```python
from build123d import *

# Parameters (mm, degrees)
F1_DEPTH = 42


with BuildPart() as f1:
    # F0 (on Right) → F1 (new body)
    with BuildSketch(Plane.YZ):
        with BuildLine():
            Line((2.25, 10), (6.75, 10))
            Line((6.75, 10), (6.75, 14.565794))
            ThreePointArc((6.75, 14.565794), (6.622824, 14.872824), (6.315794, 15))
            Line((6.315794, 15), (2.684206, 15))
            ThreePointArc((2.684206, 15), (2.377176, 14.872824), (2.25, 14.565794))
            Line((2.25, 14.565794), (2.25, 10))
        make_face()
        with BuildLine():
            Line((2.25, 5.776099), (2.25, 0.066271))
            add(Edge.make_bspline(
                [(2.25, 0.066271), (2.301244, 1.931495), (6.745765, 0.11442), (6.75, 10)],
                knots=[0.125472, 0.125472, 0.125472, 0.125472, 10.965856, 10.965856, 10.965856, 10.965856], degree=3))
            Line((6.75, 10), (2.25, 10))
            Line((2.25, 10), (2.25, 5.776099))
        make_face()
        with BuildLine():
            ThreePointArc((-2.25, -9.565794), (-2.122824, -9.872824), (-1.815794, -10))
            Line((-1.815794, -10), (1.815794, -10))
            ThreePointArc((1.815794, -10), (2.122824, -9.872824), (2.25, -9.565794))
            Line((2.25, -9.565794), (2.25, 0))
            add(Edge.make_bspline(
                [(2.25, 0), (2.249402, 0.022599), (2.249407, 0.044682), (2.25, 0.066271)],
                knots=[0, 0, 0, 0, 0.125472, 0.125472, 0.125472, 0.125472], degree=3))
            Line((2.25, 0.066271), (2.25, 5.776099))
            Line((2.25, 5.776099), (-2.25, 5.776099))
            Line((-2.25, 5.776099), (-2.25, 0.066271))
            add(Edge.make_bspline(
                [(-2.25, 0), (-2.249402, 0.022599), (-2.249407, 0.044682), (-2.25, 0.066271)],
                knots=[0, 0, 0, 0, 0.125472, 0.125472, 0.125472, 0.125472], degree=3))
            Line((-2.25, 0), (-2.25, -9.565794))
        make_face()
        with BuildLine():
            add(Edge.make_bspline(
                [(-2.25, 0.066271), (-2.301244, 1.931495), (-6.745765, 0.11442), (-6.75, 10)],
                knots=[0.125472, 0.125472, 0.125472, 0.125472, 10.965856, 10.965856, 10.965856, 10.965856], degree=3))
            Line((-2.25, 0.066271), (-2.25, 5.776099))
            Line((-2.25, 5.776099), (-2.25, 10))
            Line((-2.25, 10), (-6.75, 10))
        make_face()
        with BuildLine():
            Line((-6.75, 14.565794), (-6.75, 10))
            Line((-6.75, 10), (-2.25, 10))
            Line((-2.25, 10), (-2.25, 14.565794))
            ThreePointArc((-2.25, 14.565794), (-2.377176, 14.872824), (-2.684206, 15))
            Line((-2.684206, 15), (-6.315794, 15))
            ThreePointArc((-6.315794, 15), (-6.622824, 14.872824), (-6.75, 14.565794))
        make_face()
    extrude(amount=F1_DEPTH)


solid = f1.part
```
For this review, take the finished solid that the model builds, in its own axes (mm). A direction names the side the tool comes from. Round coordinates to 2 decimals unless told otherwise and drop trailing zeros. Write each loop counter-clockwise with the first axis right and the second up, starting at its lowest first coordinate (ties: lowest second). Pieces come first, ordered by that corner, then holes. Notation, with made-up numbers: M 35,-21.5 L 89,-21.5 A34 ccw 89,17.5 Z; hole C -21.75,69 d4. An arc over 180 degrees is marked long. One line per item, written item: value. Start each with the question number.
(1) We need section A-A (z = 12). Give the boundary of the cut face in (x, y), and give its area (3 significant figures).
(2) Wall thickness on line 1 (Y direction, x = 10.5, z = 12); line 2 (Z direction, x = 16, y = -1); line 3 (Y direction, x = 34.5, z = -4): over which ranges is each line inside the solid? List them lowest first.
(3) Insertion check: pin 1 (3 mm diameter, centred on x = 26.5, z = -6, fed in from -Y); pin 2 (8 mm diameter, centred on y = 5, z = 2.5, fed in from +X); pin 3 (1.5 mm diameter, centred on x = 37.5, z = 6.5, fed in from -Y); pin 4 (12 mm diameter, centred on x = 10.5, z = 3, fed in from -Y). Each pin has a flat end and moves straight along its axis. Give the tip position at first contact, or say it passes through.
(4) The part is to be moulded in two halves that separate along Y. For faces 1 (the flat face through (0, 0, 5)), 2 (the flat face through (21, 2.25, -5)), 3 (the flat face through (21, 0, 5.776)), say which applies: released by +Y, released by -Y, zero draft, split by the parting line, or undercut.
(5) Machinability: for faces 4 (the flat face through (21, -2.25, 10)), 5 (the flat face through (21, -2.25, -5)), 6 (the flat face through (21, 0, -10)), which of the approach directions +Z, -Z, +X, -X, +Y, -Y give a long, thin tool a straight path to every point of the face, cutting with its end or side? Answer none if there is none.
Result:
1. outline: M 0,-6.75 L 42,-6.75 L 42,-2.25 L 0,-2.25 Z; M 0,2.25 L 42,2.25 L 42,6.75 L 0,6.75 Z
1. area: 378 mm²
2. line 1: -6.75 to -2.25, 2.25 to 6.75
2. line 2: -10 to 5.78
2. line 3: -2.25 to 2.25
3. pin 1: y = -2.25
3. pin 2: x = 42
3. pin 3: y = -6.61
3. pin 4: y = -6.73
4. face 1: zero draft
4. face 2: released by +Y
4. face 3: undercut
5. face 4: +Z, +X, -X
5. face 5: -Z, +X, -X, -Y
5. face 6: -Z, +X, -X, +Y, -Y
